CAD build for the part. Positions are in the model's coordinates, mm. Face numbers are marked on the shaded views. Round coordinates to 2 decimals unless told otherwise and drop trailing zeros. Write each loop counter-clockwise with the first axis right and the second up, starting at its lowest first coordinate (ties: lowest second). Pieces come first, ordered by that corner, then holes. Notation, with made-up numbers: (-6.5, 27) - (29.5, 27) arc R6 ccw to (29.5, 31) - close; hole circle Ø6 at (54.5, 46). An arc over 180 degrees is marked (long way). Put each result on its own line as item: value. Start each with the question number.
Item 1: Mould opens along X. For the marked faces 1 and 2 say: released by +X, released by -X, zero draft, split by the parting line, or undercut.
Item 2: Pin check, flat tip, straight feed: pin 1 Ø3 at (x, z) = (52, 72) entering from -Y. Stop position of the tip, or through.
Item 3: Cut at B-B (z = 50). Give the cut face in (x, y).
Item 4: Drill centre lines: line 1 (X direction, y = 4, z = 10); line 2 (Z direction, x = 30, y = 2.25); line 3 (X direction, y = 5, z = 12). Where is each one in solid material? Low to high. Write a range as from..to.
Item 5: Cut at D-D (z = 10). Give the cut face in (x, y), and give its area (3 significant figures).
Item 6: Cut at C-C (y = 4.75). Count the separate pieces of the cut face and the enclosed holes in it, and give its area (3 significant figures).
Item 7: Cut at A-A (x = 30). Give the cut face in (y, z), and give its area (3 significant figures).
```python
from build123d import *

# Parameters (mm, degrees)
F0_R           = 24
F1_DEPTH       = 8
F2_D           = 5
F2_CSINK_D     = 10
F2_CSINK_ANGLE = 90
F3_D           = 4


with BuildPart() as f1:
    # F0 (on Front) → F1 (new body)
    with BuildSketch(Plane.XZ):
        with BuildLine():
            ThreePointArc((0, 2), (0.585786, 0.585786), (2, 0))
            Line((2, 0), (58, 0))
            ThreePointArc((58, 0), (59.414214, 0.585786), (60, 2))
            Line((60, 2), (60, 78))
            ThreePointArc((60, 78), (59.414214, 79.414214), (58, 80))
            Line((58, 80), (2, 80))
            ThreePointArc((2, 80), (0.585786, 79.414214), (0, 78))
            Line((0, 78), (0, 2))
        make_face()
        with Locations((30, 50)):
            Circle(F0_R, mode=Mode.SUBTRACT)
    extrude(amount=-F1_DEPTH)

    # F2 (through all)
    with Locations(Plane.XZ):
        with Locations((10, 10), (30, 10), (50, 10)):
            CounterSinkHole(F2_D / 2, F2_CSINK_D / 2, counter_sink_angle=F2_CSINK_ANGLE)

    # F3 (through all)
    with Locations(Plane.XZ):
        with Locations((8, 72), (52, 72), (52, 28), (8, 28)):
            Hole(F3_D / 2)


solid = f1.part
```
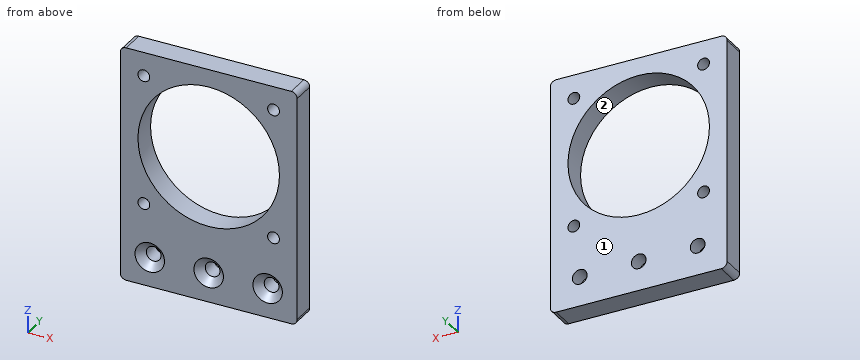
Output values:
1. face 1: zero draft
1. face 2: undercut
2. pin 1: through
3. outline: (0, 0) - (6, 0) - (6, 8) - (0, 8) - close; (54, 0) - (60, 0) - (60, 8) - (54, 8) - close
4. line 1: 0..7.5, 12.5..27.5, 32.5..47.5, 52.5..60
4. line 2: 0..7.25, 12.75..26, 74..80
4. line 3: 0..8.5, 11.5..28.5, 31.5..48.5, 51.5..60
5. outline: (0, 0) - (5, 0) - (7.5, 2.5) - (7.5, 8) - (0, 8) - close; (12.5, 2.5) - (15, 0) - (25, 0) - (27.5, 2.5) - (27.5, 8) - (12.5, 8) - close; (32.5, 2.5) - (35, 0) - (45, 0) - (47.5, 2.5) - (47.5, 8) - (32.5, 8) - close; (52.5, 2.5) - (55, 0) - (60, 0) - (60, 8) - (52.5, 8) - close
5. area: 341 mm2
6. separate pieces: 1
6. enclosed holes: 8
6. area: 2,880 mm2
7. outline: (0, 0) - (8, 0) - (8, 7.5) - (2.5, 7.5) - (0, 5) - close; (0, 15) - (2.5, 12.5) - (8, 12.5) - (8, 26) - (0, 26) - close; (0, 74) - (8, 74) - (8, 80) - (0, 80) - close
7. area: 210 mm2
